```python
from build123d import *

# Parameters (mm, degrees)
F1_DEPTH = 609.6
F3_DEPTH = 79.443993
F5_DEPTH = 79.443993
F6_R     = 19.05


with BuildPart() as f1:
    # F0 (on Front) → F1 (new body)
    with BuildSketch(Plane.XZ):
        Polygon((5.433592, 55.333211), (-102.516408, 55.333211), (-102.516408, 48.983211), (0, 48.983211), (0, -24.109783), (6.349577, -24.036504), align=None)
    extrude(amount=F1_DEPTH)

    # F2 (on face) → F3 (cut, through all)
    with BuildSketch(Plane.XY.offset(55.333211)):
        with BuildLine():
            Line((-32.666408, -46.241132), (-88.546408, -46.241132))
            ThreePointArc((-88.546408, -46.241132), (-93.105277, -50.8), (-88.546408, -55.358868))
            Line((-88.546408, -55.358868), (-32.666408, -55.358868))
            ThreePointArc((-32.666408, -55.358868), (-28.10754, -50.8), (-32.666408, -46.241132))
        make_face()
        with BuildLine():
            Line((-32.666408, -554.241132), (-88.546408, -554.241132))
            ThreePointArc((-88.546408, -554.241132), (-93.105277, -558.8), (-88.546408, -563.358868))
            Line((-88.546408, -563.358868), (-32.666408, -563.358868))
            ThreePointArc((-32.666408, -563.358868), (-28.10754, -558.8), (-32.666408, -554.241132))
        make_face()
    extrude(amount=-F3_DEPTH, mode=Mode.SUBTRACT)

    # F4 (on face) → F5 (cut, through all)
    with BuildSketch(Plane.XY.offset(55.333211)):
        with BuildLine():
            Line((-26.316408, -426.085), (-88.546408, -426.085))
            ThreePointArc((-88.546408, -426.085), (-94.261408, -431.8), (-88.546408, -437.515))
            Line((-88.546408, -437.515), (-26.316408, -437.515))
            ThreePointArc((-26.316408, -437.515), (-20.601408, -431.8), (-26.316408, -426.085))
        make_face()
    extrude(amount=-F5_DEPTH, mode=Mode.SUBTRACT)

    # F6
    f6_edges = [f1.edges().sort_by_distance(p)[0] for p in [
        (3.174789, -609.6, -24.073143),
        (3.174789, 0, -24.073143),
    ]]
    fillet(f6_edges, radius=F6_R)


solid = f1.part
```
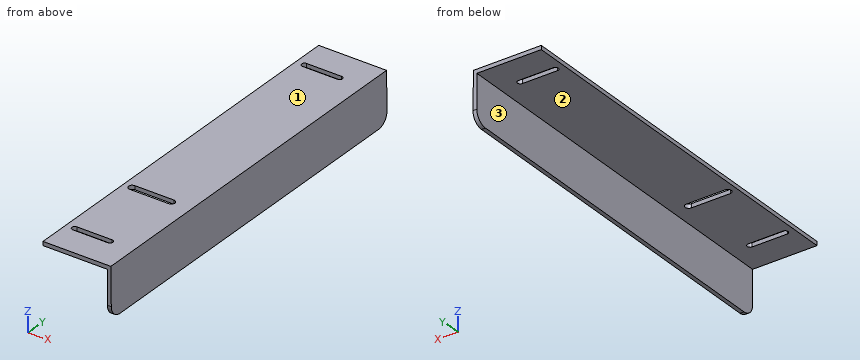
Verification items for the finished model (mm, model axes). Face numbers are marked on the shaded views. Give positions to 0.01 mm unless a question says otherwise; leave off trailing zeros. Order: outer loops, then holes, each group sorted by start corner. A loop starts at its lowest first (then second) coordinate and runs counter-clockwise, first axis right, second up. Notation, with made-up numbers: (-19, 84.5) - (5, 84.5) arc R18 cw to (5, 90.5) - close; hole circle Ø7 at (52.25, 22.25). An arc over 180 degrees is marked (long way). Answer as CSV lines item,"result". Start each with the question number.
Item 1: Mould release check, pull along Z, two halves, no side actions. Record for the marked faces 1, 2 and 3: released by +Z, released by -Z, zero draft, split by the parting line, or undercut.
Item 2: Section check A-A, the plane x = -78. Record the boundary of the cut face in (y, z) (3 decimals), plus the area to 3 significant figures.
Item 3: Gauge pin test, flat ends, axial feed: pin 1 (1.5 mm diameter, centred on x = -44.5, y = -266.5, fed in from -Z); pin 2 (1 mm diameter, centred on y = -332, z = 22.5, fed in from -X); pin 3 (8 mm diameter, centred on y = -142.5, z = 43, fed in from +X). Record the tip position at first contact, or that the pin passes through.
Item 4: Section check C-C, the plane y = -73.5. Record the boundary of the cut face in (x, z), plus the area to 3 significant figures.
Item 5: Section check D-D, the plane x = -8. Record the boundary of the cut face in (y, z).
Item 6: Section check B-B, the plane y = -431.8. Record the boundary of the cut face in (x, z).
Item 7: Material ranges on L1, parallel to Z at x = -92, y = -566.5; L2, parallel to X at y = -165, z = 45; L3, parallel to X at y = -127, z = 46.5, recorded low to high.
Filled in:
1,face 1,"released by +Z"
1,face 2,"released by -Z"
1,face 3,"zero draft"
2,outline,"(-609.6, 48.983) - (-563.359, 48.983) - (-563.359, 55.333) - (-609.6, 55.333) - close; (-554.241, 48.983) - (-437.515, 48.983) - (-437.515, 55.333) - (-554.241, 55.333) - close; (-426.085, 48.983) - (-55.359, 48.983) - (-55.359, 55.333) - (-426.085, 55.333) - close; (-46.241, 48.983) - (0, 48.983) - (0, 55.333) - (-46.241, 55.333) - close"
2,area,"3,680 mm^2"
3,pin 1,"z = 48.98"
3,pin 2,"x = 0"
3,pin 3,"x = 5.62"
4,outline,"(-102.52, 48.98) - (0, 48.98) - (0, -24.11) - (6.35, -24.04) - (5.43, 55.33) - (-102.52, 55.33) - close"
4,area,"1,120 mm^2"
5,outline,"(-609.6, 48.98) - (0, 48.98) - (0, 55.33) - (-609.6, 55.33) - close"
6,outline,"(-102.52, 48.98) - (-94.26, 48.98) - (-94.26, 55.33) - (-102.52, 55.33) - close; (-20.6, 48.98) - (0, 48.98) - (0, -24.11) - (6.35, -24.04) - (5.43, 55.33) - (-20.6, 55.33) - close"
7,L1,"48.98 to 55.33"
7,L2,"0 to 5.55"
7,L3,"0 to 5.54"
